Read the model definition and answer for the solid it produces. Units are mm, in the model's axes. A direction names the side the tool comes from. Round coordinates to 2 decimals unless told otherwise and drop trailing zeros. Write each loop counter-clockwise with the first axis right and the second up, starting at its lowest first coordinate (ties: lowest second). Pieces come first, ordered by that corner, then holes. Notation, with made-up numbers: (76.5, -23) - (109.5, -23) arc R21 ccw to (109.5, -4) - close; hole circle Ø8 at (64, 14.5). An arc over 180 degrees is marked (long way). Answer as CSV lines item,"result". Start each with the question number.
1) Find section D-D on z = -99.5. Determine the outline of the cut face in (x, y), then the cut area to 3 significant figures.
2) Find section B-B on x = 46. Determine the outline of the cut face in (y, z), then the cut area to 3 significant figures.
3) Each of these flat-tipped pins is pushed along its axis until it touches: pin 1 (1.5 mm diameter, centred on x = -44.5, y = 2, fed in from +Z); pin 2 (0.9 mm diameter, centred on x = 86, y = 1.5, fed in from -Z); pin 3 (1.5 mm diameter, centred on x = -23, y = 2, fed in from -Z); pin 4 (12 mm diameter, centred on x = 64.5, z = -252.5, fed in from +Y). Where does it stop, or does it pass through?
4) Find section A-A on z = -171. Determine the outline of the cut face in (x, y).
5) Find section C-C on y = 1.9. State how many separate pieces and enclosed holes the cut face has, then the cut area to 3 significant figures.
6) Consider line 1 along Z through (x, y) = (27, 0.7); line 2 along Z through (x, y) = (-17, 0.5); line 3 along Z through (x, y) = (74.5, 0.8). Determine where each line is inside the solid, lowest interval first.
7) Which of the six approach directions +Z, -Z, +X, -X, +Y, -Y give full straight-line access (tool end or side, diameter ignored) to faces 4 (the cylindrical face through (95.2, 1.5, 14.7)), 5 (the cylindrical face through (-38.73, 1.52, -199.48))?
8) For a pull along Z with two mould halves and no side action, classify faces 1 (the cylindrical face through (-38.605, 1.521, -133.794)), 2 (the cylindrical face through (-46.803, 1.479, -348.145)), 3 (the flat face through (23, 0, -127)) as +Z half, -Z half, draft (parallel to the pull), parting line (faces both ways), or undercut.
from build123d import *

# Parameters (mm, degrees)
RESSALTO_EXTRUS_O1_DEPTH = 3
ESBO_O2_R                = 1.5
ESBO_O2_W                = 3
ESBO_O2_H                = 10
ESBO_O2_W_2              = 10
ESBO_O2_H_2              = 3
ESBO_O2_H_3              = 10.102691272
CORTE_EXTRUS_O2_DEPTH    = 3


with BuildPart() as part:
    # Esboço1 → Ressalto-extrusão1 (new body)
    with BuildSketch(Plane(origin=(0, 0, 0), x_dir=(1, 0, 0), z_dir=(0, 1, 0))):
        with BuildLine():
            Line((-25.82411142, -23.300209544), (74.17588858, -23.300209544))
            ThreePointArc((74.17588858, -23.300209544), (95.389092016, -14.513412979), (104.17588858, 6.699790456))
            Line((104.17588858, 6.699790456), (104.17588858, 36.699790456))
            Line((104.17588858, 36.699790456), (64.17588858, 36.699790456))
            Line((64.17588858, 36.699790456), (64.17588858, 116.699790456))
            Line((64.17588858, 116.699790456), (104.17588858, 116.699790456))
            Line((104.17588858, 116.699790456), (104.17588858, 216.699790456))
            Line((104.17588858, 216.699790456), (64.17588858, 216.699790456))
            Line((64.17588858, 216.699790456), (64.17588858, 296.699790456))
            Line((64.17588858, 296.699790456), (104.17588858, 296.699790456))
            Line((104.17588858, 296.699790456), (104.17588858, 326.699790456))
            ThreePointArc((104.17588858, 326.699790456), (95.389092016, 347.912993892), (74.17588858, 356.699790456))
            Line((74.17588858, 356.699790456), (-25.82411142, 356.699790456))
            ThreePointArc((-25.82411142, 356.699790456), (-47.037314855, 347.912993892), (-55.82411142, 326.699790456))
            Line((-55.82411142, 326.699790456), (-55.82411142, 296.699790456))
            Line((-55.82411142, 296.699790456), (-15.82411142, 296.699790456))
            Line((-15.82411142, 296.699790456), (-15.82411142, 216.699790456))
            Line((-15.82411142, 216.699790456), (-55.82411142, 216.699790456))
            Line((-55.82411142, 216.699790456), (-55.82411142, 116.699790456))
            Line((-55.82411142, 116.699790456), (-15.82411142, 116.699790456))
            Line((-15.82411142, 116.699790456), (-15.82411142, 36.699790456))
            Line((-15.82411142, 36.699790456), (-55.82411142, 36.699790456))
            Line((-55.82411142, 36.699790456), (-55.82411142, 6.699790456))
            ThreePointArc((-55.82411142, 6.699790456), (-47.037314855, -14.513412979), (-25.82411142, -23.300209544))
        make_face()
    extrude(amount=RESSALTO_EXTRUS_O1_DEPTH)

    # Esboço2 → Corte-extrusão2 (cut)
    with BuildSketch(Plane(origin=(0, 3, 0), x_dir=(1, 0, 0), z_dir=(0, 1, 0))):
        with Locations(Location((-44.32411142, 205.199790456, 0), (0, 0, 270))):
            Circle(ESBO_O2_R)
        with Locations(Location((-44.32411142, 128.199790456, 0), (0, 0, 270))):
            Circle(ESBO_O2_R)
        with Locations(Location((92.67588858, 128.199790456, 0), (0, 0, 270))):
            Circle(ESBO_O2_R)
        with Locations(Location((92.67588858, 205.199790456, 0), (0, 0, 270))):
            Circle(ESBO_O2_R)
        with Locations((102.67588858, 321.699790456)):
            Rectangle(ESBO_O2_W, ESBO_O2_H)
        with Locations((69.17588858, 355.199790456)):
            Rectangle(ESBO_O2_W_2, ESBO_O2_H_2)
        with BuildLine():
            Line((-36.32411142, 205.199790456), (84.67588858, 205.199790456))
            ThreePointArc((84.67588858, 205.199790456), (87.019034331, 199.542936207), (92.67588858, 197.199790456))
            Line((92.67588858, 197.199790456), (92.67588858, 136.199790456))
            ThreePointArc((92.67588858, 136.199790456), (87.019034331, 133.856644706), (84.67588858, 128.199790456))
            Line((84.67588858, 128.199790456), (-36.32411142, 128.199790456))
            ThreePointArc((-36.32411142, 128.199790456), (-38.66725717, 133.856644706), (-44.32411142, 136.199790456))
            Line((-44.32411142, 136.199790456), (-44.32411142, 197.199790456))
            ThreePointArc((-44.32411142, 197.199790456), (-38.66725717, 199.542936207), (-36.32411142, 205.199790456))
        make_face()
        with Locations((-14.32411142, 1.699790456)):
            Rectangle(ESBO_O2_W, ESBO_O2_H)
        with Locations((62.67588858, 1.64844482)):
            Rectangle(ESBO_O2_W, ESBO_O2_H_3)
        with Locations((-20.82411142, 355.199790456)):
            Rectangle(ESBO_O2_W_2, ESBO_O2_H_2)
        with Locations((-54.32411142, 321.699790456)):
            Rectangle(ESBO_O2_W, ESBO_O2_H)
        Polygon((34.10088858, 256.699790456), (34.10088858, 266.099790456), (14.25088858, 266.099790456), (14.25088858, 256.699790456), (14.25088858, 226.099790456), (34.10088858, 226.099790456), align=None)
    extrude(amount=-CORTE_EXTRUS_O2_DEPTH, mode=Mode.SUBTRACT)


solid = part.part
Check values:
1,outline,"(-15.82, 0) - (64.18, 0) - (64.18, 3) - (-15.82, 3) - close"
1,area,"240 mm^2"
2,outline,"(0, -356.7) - (3, -356.7) - (3, -205.2) - (0, -205.2) - close; (0, -128.2) - (3, -128.2) - (3, 23.3) - (0, 23.3) - close"
2,area,"909 mm^2"
3,pin 1,"stops at z = 17.36"
3,pin 2,"stops at z = -354.46"
3,pin 3,"stops at z = -353.7"
3,pin 4,"stops at y = 3"
4,outline,"(-55.82, 0) - (-44.32, 0) - (-44.32, 3) - (-55.82, 3) - close; (92.68, 0) - (104.18, 0) - (104.18, 3) - (92.68, 3) - close"
5,separate pieces,"1"
5,enclosed holes,"8"
5,area,"35,900 mm^2"
6,line 1,"z = -356.7 to -266.1, -226.1 to -205.2, -128.2 to 23.3"
6,line 2,"z = -353.7 to -296.7, -216.7 to -205.2, -128.2 to -116.7, -36.7 to 23.3"
6,line 3,"z = -356.7 to -296.7, -216.7 to -205.2, -128.2 to -116.7, -36.7 to 23.3"
7,face 4,"+Z, +X, +Y, -Y"
7,face 5,"+Y, -Y"
8,face 1,"undercut"
8,face 2,"-Z half"
8,face 3,"draft"
